Here's how the part is built. I have some questions about the finished solid (model axes, mm). Face numbers are marked on the shaded views. A direction names the side the tool comes from. Round coordinates to 2 decimals unless told otherwise and drop trailing zeros. Order: outer loops, then holes, each group sorted by start corner. A loop starts at its lowest first (then second) coordinate and runs counter-clockwise, first axis right, second up. Notation, with made-up numbers: (-11, 14) - (41, 14) arc R35 ccw to (41, 46) - close; hole circle Ø7 at (-29.75, -27.5). An arc over 180 degrees is marked (long way). Answer as a JSON object with one key per item and string values.
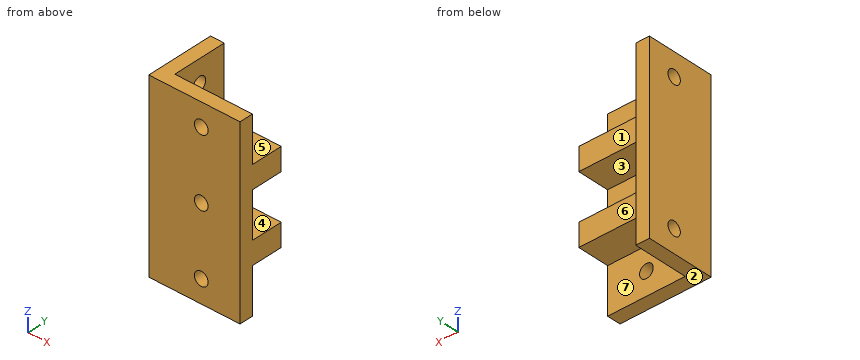
```python
from build123d import *

# Parameters (mm, degrees)
EXTRUDE_1_DEPTH     = 40
SKETCH_3_R          = 1.5
CUT_EXTRUDE_1_DEPTH = 46.97825573
SKETCH_4_R          = 1.5
CUT_EXTRUDE_2_DEPTH = 47.303347611
SKETCH_5_W          = 17
SKETCH_5_H          = 5
EXTRUDE_2_DEPTH     = 7


with BuildPart() as part:
    # 草图1 → 凸台-拉伸1 (new body)
    with BuildSketch(Plane.XY):
        Polygon((0, 0), (0, 15), (3, 15), (3, 3), (20, 3), (20, 0), align=None)
    extrude(amount=EXTRUDE_1_DEPTH)

    # 草图3 → 切除-拉伸1 (cut, through all)
    with BuildSketch(Plane(origin=(3, 0, 0), x_dir=(0, 0, -1), z_dir=(1, 0, 0))):
        with Locations(Location((-35, 9, 0), (0, 0, 90))):
            Circle(SKETCH_3_R)
        with Locations(Location((-5, 9, 0), (0, 0, 270))):
            Circle(SKETCH_3_R)
    extrude(amount=-CUT_EXTRUDE_1_DEPTH, mode=Mode.SUBTRACT)

    # 草图4 → 切除-拉伸2 (cut, through all)
    with BuildSketch(Plane(origin=(0, 3, 0), x_dir=(1, 0, 0), z_dir=(0, 1, 0))):
        with Locations(Location((11.5, -20, 0), (0, 0, 270))):
            Circle(SKETCH_4_R)
        with Locations(Location((11.5, -35, 0), (0, 0, 270))):
            Circle(SKETCH_4_R)
        with Locations(Location((11.5, -5, 0), (0, 0, 90))):
            Circle(SKETCH_4_R)
    extrude(amount=-CUT_EXTRUDE_2_DEPTH, mode=Mode.SUBTRACT)

    # 草图5 → 凸台-拉伸2 (add)
    with BuildSketch(Plane(origin=(0, 3, 0), x_dir=(1, 0, 0), z_dir=(0, 1, 0))):
        with Locations((11.5, -27.5)):
            Rectangle(SKETCH_5_W, SKETCH_5_H)
        with Locations((11.5, -12.5)):
            Rectangle(SKETCH_5_W, SKETCH_5_H)
    extrude(amount=EXTRUDE_2_DEPTH)


solid = part.part
```
1. If I drill on L1, parallel to Z at x = 17.75, y = 7.5; L2, parallel to X at y = 0.8, z = 35; L3, parallel to Z at x = 2.5, y = 8.75, over which ranges is the centre line in solid material (lowest first)? Write a range as [from, to].
Responses:
{"L1": "[10, 15], [25, 30]", "L2": "[0, 10], [13, 20]", "L3": "[0, 3.52], [6.48, 33.52], [36.48, 40]"}
2. Imagine slicing it at B-B (y = 9). List the corners of the cut face in (x, z) for me.
Responses:
{"outline": "(0, 0) - (3, 0) - (3, 3.5) - (0, 3.5) - close; (0, 6.5) - (3, 6.5) - (3, 10) - (20, 10) - (20, 15) - (3, 15) - (3, 25) - (20, 25) - (20, 30) - (3, 30) - (3, 33.5) - (0, 33.5) - close; (0, 36.5) - (3, 36.5) - (3, 40) - (0, 40) - close"}
3. Imagine slicing it at A-A (z = 20). List the corners of the cut face in (x, y) for me, plus the area to 3 significant figures.
Responses:
{"outline": "(0, 0) - (10, 0) - (10, 3) - (3, 3) - (3, 15) - (0, 15) - close; (13, 0) - (20, 0) - (20, 3) - (13, 3) - close", "area": "87.0 mm2"}
4. For the marked faces 4, 5, 6 and 7, which set-ups out of +Z, -Z, +X, -X, +Y, -Y let a thin tool reach every point of the face, with its end or its side?
Responses:
{"face 4": "+X, +Y", "face 5": "+Z, +X, +Y", "face 6": "+Z, -Z, +X, +Y", "face 7": "-Z, +X, +Y"}
5. For P1, Ø4, axis at y = 9, z = 35, coming from the +X side; P2, Ø5, axis at x = 9.5, y = 10, coming from the -Z side; P3, Ø5, axis at x = 12, z = 19, coming from the +Y side, each with a flat end and sliding along its axis, tell me the tip position at first contact or that it passes through.
Responses:
{"P1": "x = 3", "P2": "z = 10", "P3": "y = 3"}
6. Thinking about a two-plate mould opening in Z: for the marked faces 1, 2 and 3, which applies, pulls with the +Z half, pulls with the -Z half, needs draft (parallel to the pull), parting line crosses it, or undercut?
Responses:
{"face 1": "needs draft", "face 2": "pulls with the -Z half", "face 3": "undercut"}
7. Imagine slicing it at D-D (z = 35). List the corners of the cut face in (x, y) for me, plus the area to 3 significant figures.
Responses:
{"outline": "(0, 0) - (10, 0) - (10, 3) - (3, 3) - (3, 7.5) - (0, 7.5) - close; (0, 10.5) - (3, 10.5) - (3, 15) - (0, 15) - close; (13, 0) - (20, 0) - (20, 3) - (13, 3) - close", "area": "78.0 mm2"}
8. Imagine slicing it at C-C (x = 11.5). List the corners of the cut face in (y, z) for me.
Responses:
{"outline": "(0, 0) - (3, 0) - (3, 3.5) - (0, 3.5) - close; (0, 6.5) - (3, 6.5) - (3, 10) - (10, 10) - (10, 15) - (3, 15) - (3, 18.5) - (0, 18.5) - close; (0, 21.5) - (3, 21.5) - (3, 25) - (10, 25) - (10, 30) - (3, 30) - (3, 33.5) - (0, 33.5) - close; (0, 36.5) - (3, 36.5) - (3, 40) - (0, 40) - close"}
